Design review of the part built by this model. Coordinates are the model's own, in mm. Face numbers are marked on the shaded views. A direction names the side the tool comes from. Round coordinates to 2 decimals unless told otherwise and drop trailing zeros. Write each loop counter-clockwise with the first axis right and the second up, starting at its lowest first coordinate (ties: lowest second). Pieces come first, ordered by that corner, then holes. Notation, with made-up numbers: (13, -40) - (43, -40) arc R24 ccw to (43, -17) - close; hole circle Ø11 at (60.5, 88). An arc over 180 degrees is marked (long way). Use one line per item in the form item = value.
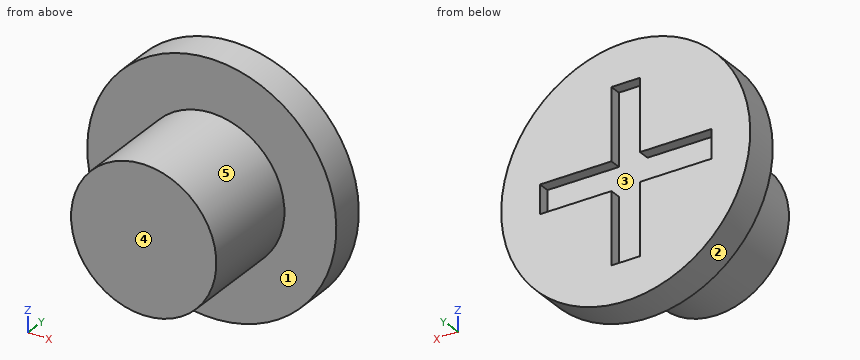
```python
from build123d import *

# Parameters (mm, degrees)
SKETCH1_R           = 3.175
BOSS_EXTRUDE1_DEPTH = 21.54
SKETCH2_R           = 5.442868
BOSS_EXTRUDE2_DEPTH = 1.5
SKETCH3_W           = 1.25
SKETCH3_H           = 3.125
SKETCH3_W_2         = 3.125
SKETCH3_H_2         = 1.25
CUT_EXTRUDE2_DEPTH  = 0.5
SKETCH4_R           = 3.175
CUT_EXTRUDE3_DEPTH  = 17


with BuildPart() as part:
    # Sketch1 → Boss-Extrude1 (new body)
    with BuildSketch(Plane(origin=(0, 0, 0), x_dir=(1, 0, 0), z_dir=(0, 1, 0))):
        with Locations(Location((0, 0, 0), (0, 0, 270))):
            Circle(SKETCH1_R)
    extrude(amount=BOSS_EXTRUDE1_DEPTH)

    # Sketch2 → Boss-Extrude2 (add)
    with BuildSketch(Plane(origin=(0, 21.54, 0), x_dir=(1, 0, 0), z_dir=(0, 1, 0))):
        with Locations(Location((0, 0, 0), (0, 0, 270))):
            Circle(SKETCH2_R)
    extrude(amount=BOSS_EXTRUDE2_DEPTH)

    # Sketch3 → Cut-Extrude2 (cut)
    with BuildSketch(Plane(origin=(0, 23.04, 0), x_dir=(1, 0, 0), z_dir=(0, 1, 0))):
        with Locations((0, -2.1875)):
            Rectangle(SKETCH3_W, SKETCH3_H)
        with Locations((-2.1875, 0)):
            Rectangle(SKETCH3_W_2, SKETCH3_H_2)
        with Locations((0, 2.1875)):
            Rectangle(SKETCH3_W, SKETCH3_H)
        with Locations((2.1875, 0)):
            Rectangle(SKETCH3_W_2, SKETCH3_H_2)
        Rectangle(SKETCH3_W, SKETCH3_H_2)
    extrude(amount=-CUT_EXTRUDE2_DEPTH, mode=Mode.SUBTRACT)

    # Sketch4 → Cut-Extrude3 (cut)
    with BuildSketch(Plane.XZ):
        with Locations(Location((0, 0, 0), (0, 0, 270))):
            Circle(SKETCH4_R)
    extrude(amount=-CUT_EXTRUDE3_DEPTH, mode=Mode.SUBTRACT)


solid = part.part
```
Q1. To check wall thickness, follow line 1 along Y through (x, z) = (4.5, 0); line 2 along Y through (x, z) = (-3.25, 0); line 3 along X through (y, z) = (17.5, -2.5). State the ranges of each line that lie inside material, in increasing order. Write a range as from..to.
Calculated:
line_1 = 21.54..23.04
line_2 = 21.54..22.54
line_3 = -1.96..1.96
Q2. We need section A-A on x = 0. Write out the cut boundary in (y, z) (3 decimals).
Calculated:
outline = (17, -3.175) - (21.54, -3.175) - (21.54, -5.443) - (23.04, -5.443) - (23.04, -3.75) - (22.54, -3.75) - (22.54, 3.75) - (23.04, 3.75) - (23.04, 5.443) - (21.54, 5.443) - (21.54, 3.175) - (17, 3.175) - close
Q3. Machinability: for the marked faces 4 and 5, which of the approach directions +Z, -Z, +X, -X, +Y, -Y give a long, thin tool a straight path to every point of the face, cutting with its end or side? Answer none if there is none.
Calculated:
face_4 = +Z, -Z, +X, -X, -Y
face_5 = -Y
Q4. We need section C-C on y = 18.25. Write out the cut boundary in (x, z) (3 decimals).
Calculated:
outline = circle Ø6.35 at (0, 0)
Q5. We need section D-D on z = -3.5. Write out the cut boundary in (x, y) (3 decimals), then the cut area to 3 significant figures.
Calculated:
outline = (-4.168, 21.54) - (4.168, 21.54) - (4.168, 23.04) - (0.625, 23.04) - (0.625, 22.54) - (-0.625, 22.54) - (-0.625, 23.04) - (-4.168, 23.04) - close
area = 11.9 mm2
Q6. We need section B-B on z = -1.5. Write out the cut boundary in (x, y) (3 decimals), then the cut area to 3 significant figures.
Calculated:
outline = (-5.232, 21.54) - (-2.798, 21.54) - (-2.798, 17) - (2.798, 17) - (2.798, 21.54) - (5.232, 21.54) - (5.232, 23.04) - (0.625, 23.04) - (0.625, 22.54) - (-0.625, 22.54) - (-0.625, 23.04) - (-5.232, 23.04) - close
area = 40.5 mm2
Q7. Draft analysis for pull direction Z (two halves, no side actions). For the marked faces 1, 2 and 3, state which applies: released by +Z, released by -Z, zero draft, split by the parting line, or undercut.
Calculated:
face_1 = zero draft
face_2 = split by the parting line
face_3 = undercut
Q8. For P1, Ø3, axis at y = 20.5, z = -2, coming from the -X side; P2, Ø1, axis at y = 20, z = -4.5, coming from the +X side, all flat-tipped, find the tip position at first contact; note any pin that passes through.
Calculated:
P1 = -5.36
P2 = through
